Geometry check sheet. Reference: the model listing, model coordinates, mm. A direction names the side the tool comes from. Coordinates: 2 decimals unless noted, no trailing zeros. Order: outer loops, then holes, each group sorted by start corner. A loop starts at its lowest first (then second) coordinate and runs counter-clockwise, first axis right, second up. Notation, with made-up numbers: (5.5, 33) - (11.5, 33) arc R22 cw to (11.5, 61) - close; hole circle Ø8 at (75.25, 85.5). An arc over 180 degrees is marked (long way). Put each result on its own line as item: value.
from build123d import *

# Parameters (mm, degrees)
SKETCH1_R           = 1
SKETCH1_W           = 2.92
SKETCH1_H           = 2.92
BOSS_EXTRUDE1_DEPTH = 3


with BuildPart() as part:
    # Sketch1 → Boss-Extrude1 (new body)
    with BuildSketch(Plane.XY):
        Polygon((-16.517509728, 23.247171726), (-16.517509728, 26.247171726), (-26.517509728, 26.247171726), (-26.517509728, 23.247171726), (-31.517509728, 23.247171726), (-31.517509728, 18.247171726), (-34.517509728, 18.247171726), (-34.517509728, 8.247171726), (-31.517509728, 8.247171726), (-31.517509728, -1.752828274), (-39.517509728, -1.752828274), (-39.517509728, -11.752828274), (-31.517509728, -11.752828274), (-31.517509728, -21.752828274), (-34.517509728, -21.752828274), (-34.517509728, -31.752828274), (-31.517509728, -31.752828274), (-31.517509728, -36.752828274), (-26.517509728, -36.752828274), (-26.517509728, -39.752828274), (-16.517509728, -39.752828274), (-16.517509728, -36.752828274), (-6.517509728, -36.752828274), (-6.517509728, -44.752828274), (3.482490272, -44.752828274), (3.482490272, -36.752828274), (13.482490272, -36.752828274), (13.482490272, -39.752828274), (23.482490272, -39.752828274), (23.482490272, -36.752828274), (28.482490272, -36.752828274), (28.482490272, -31.752828274), (31.482490272, -31.752828274), (31.482490272, -21.752828274), (28.482490272, -21.752828274), (28.482490272, -11.752828274), (36.482490272, -11.752828274), (36.482490272, -1.752828274), (28.482490272, -1.752828274), (28.482490272, 8.247171726), (31.482490272, 8.247171726), (31.482490272, 18.247171726), (28.482490272, 18.247171726), (28.482490272, 23.247171726), (23.482490272, 23.247171726), (23.482490272, 26.247171726), (13.482490272, 26.247171726), (13.482490272, 23.247171726), (3.482490272, 23.247171726), (3.482490272, 31.247171726), (-6.517509728, 31.247171726), (-6.517509728, 23.247171726), align=None)
        with Locations((-22.517509728, -33.752828274)):
            Circle(SKETCH1_R, mode=Mode.SUBTRACT)
        with Locations((5.482490272, -33.752828274)):
            Circle(SKETCH1_R, mode=Mode.SUBTRACT)
        with Locations((-27.517509728, 19.747171726)):
            Circle(SKETCH1_R, mode=Mode.SUBTRACT)
        with Locations((20.482490272, 17.747171726)):
            Circle(SKETCH1_R, mode=Mode.SUBTRACT)
        with Locations((-1.517509728, 27.707171726)):
            Rectangle(SKETCH1_W, SKETCH1_H, mode=Mode.SUBTRACT)
        with Locations((-35.977509728, -6.752828274)):
            Rectangle(SKETCH1_W, SKETCH1_H, mode=Mode.SUBTRACT)
        with Locations((32.942490272, -6.752828274)):
            Rectangle(SKETCH1_W, SKETCH1_H, mode=Mode.SUBTRACT)
        with Locations((-1.517509728, -41.212828274)):
            Rectangle(SKETCH1_W, SKETCH1_H, mode=Mode.SUBTRACT)
    extrude(amount=BOSS_EXTRUDE1_DEPTH)


solid = part.part
Q1. Thickness scan on L1, parallel to Y at x = -1, z = 1.8; L2, parallel to X at y = -37, z = 2.2; L3, parallel to Y at x = -33.5, z = 0.55. Record the ranges inside material, lowest first. Write a range as [from, to].
Answer block:
L1: y = [-44.75, -42.67], [-39.75, 26.25], [29.17, 31.25]
L2: x = [-26.52, -16.52], [-6.52, 3.48], [13.48, 23.48]
L3: y = [-31.75, -21.75], [-11.75, -1.75], [8.25, 18.25]
Q2. Depth check by flat-ended pin: pin 1 Ø0.9 at (x, z) = (-21, 1.5) entering from +Y; pin 2 Ø5 at (x, y) = (6.5, 11.5) entering from -Z; pin 3 Ø1.5 at (y, z) = (25, 1) entering from -X; pin 4 Ø0.9 at (y, z) = (-34, 1.5) entering from +X. Enter the tip coordinate at first touch or a pass-through.
Answer block:
pin 1: stops at y = 26.25
pin 2: stops at z = 0
pin 3: stops at x = -26.52
pin 4: stops at x = 28.48
Q3. Draft check along Y on faces 1 (the flat face through (-6.518, 27, 1)), 2 (the flat face through (-22, -39.753, 1)), 3 (the flat face through (-33, 8.247, 1)), 4 (the flat face through (-34.518, -7, 1)). Enter one of: pulls with the +Y half, pulls with the -Y half, needs draft (parallel to the pull), parting line crosses it, or undercut.
Answer block:
face 1: needs draft
face 2: pulls with the -Y half
face 3: undercut
face 4: undercut
Q4. Section check D-D on z = 2.25. State how many separate pieces and enclosed holes the cut face has, then the cut area to 3 significant figures.
Answer block:
separate pieces: 1
enclosed holes: 8
area: 4,110 mm^2
Q5. Access from +Z, -Z, +X, -X, +Y, -Y to the whole of each face (thin tool, end or side, straight path). Record for faces 5 (the flat face through (-31.518, -34, 1)), 6 (the flat face through (23.482, 25, 1)), 7 (the flat face through (-36, -11.753, 1)), 8 (the flat face through (-21, 26.247, 1)).
Answer block:
face 5: +Z, -Z, -X, -Y
face 6: +Z, -Z, +X, +Y
face 7: +Z, -Z, -X
face 8: +Z, -Z, -X, +Y
Q6. Section check C-C on y = 2. Record the boundary of the cut face in (x, z), then the cut area to 3 significant figures.
Answer block:
outline: (-31.52, 0) - (28.48, 0) - (28.48, 3) - (-31.52, 3) - close
area: 180 mm^2
Q7. Section check A-A on y = -7. Record the boundary of the cut face in (x, z).
Answer block:
outline: (-39.52, 0) - (-37.44, 0) - (-37.44, 3) - (-39.52, 3) - close; (-34.52, 0) - (31.48, 0) - (31.48, 3) - (-34.52, 3) - close; (34.4, 0) - (36.48, 0) - (36.48, 3) - (34.4, 3) - close
Q8. Section check B-B on x = 25. Record the boundary of the cut face in (y, z), then the cut area to 3 significant figures.
Answer block:
outline: (-36.75, 0) - (23.25, 0) - (23.25, 3) - (-36.75, 3) - close
area: 180 mm^2
